Can you work these out from the model? Positions are in its coordinate system, mm. Give positions to 0.01 mm unless a question says otherwise; leave off trailing zeros. Order: outer loops, then holes, each group sorted by start corner. A loop starts at its lowest first (then second) coordinate and runs counter-clockwise, first axis right, second up. Notation, with made-up numbers: M -2.5,47 L 42.5,47 A23 ccw 42.5,78 Z; hole C 36.5,-21 d10. An arc over 180 degrees is marked long. One line per question, with ' | ' between items. Start each with the question number.
1) If we section it at A-A, the plane x = 0.7: State how many separate pieces and enclosed holes the cut face has, plus the area to 3 significant figures.
2) Please list where these lines run through material, in increasing order: line 1 along Z through (x, y) = (1.5, 95.25) (3 decimals); line 2 along Y through (x, z) = (1.35, 0) (3 decimals); line 3 along Z through (x, y) = (1.2, 104.75) (3 decimals). Write a range as [from, to].
3) If we section it at B-B, the plane z = -34.5: Please give me the cut outline in (x, y) (3 decimals).
4) I'm going to push flat-ended pins straight in: pin 1 Ø3.5 at (y, z) = (95.25, 9.5) entering from -X; pin 2 Ø1.6 at (x, y) = (1, 98.5) entering from +Z (3 decimals); pin 3 Ø1.6 at (x, z) = (1, 43) entering from -Y; pin 4 Ø1.6 at (x, z) = (1.5, 45) entering from +Y. Where does each tip first touch, or does it pass through?
```python
from build123d import *

# Parameters (mm, degrees)
SKETCH1_W               = 95.25
SKETCH1_H               = 311.15
BOSS_EXTRUDE1_DEPTH     = 3.175
SKETCH2_W               = 12.7
SKETCH2_H               = 3.175
SKETCH2_W_2             = 19.05
CUT_EXTRUDE1_DEPTH      = 3.175
SKETCH3_W               = 6.35
SKETCH3_H               = 10.16
CUT_EXTRUDE2_DEPTH      = 3.175
MIRROR3_COPY_1_SKETCH_W = 6.35
MIRROR3_COPY_1_SKETCH_H = 10.16
MIRROR3_COPY_1_DEPTH    = 3.175
CUT_EXTRUDE3_DEPTH      = 3.175


with BuildPart() as part:
    # Sketch1 → Boss-Extrude1 (new body)
    with BuildSketch(Plane(origin=(0, 0, 0), x_dir=(0, 0, -1), z_dir=(1, 0, 0))):
        Rectangle(SKETCH1_W, SKETCH1_H)
    extrude(amount=BOSS_EXTRUDE1_DEPTH)

    # Sketch2 → Cut-Extrude1 (cut)
    with BuildSketch(Plane(origin=(3.175, 0, 0), x_dir=(0, 0, -1), z_dir=(1, 0, 0))):
        with Locations((9.525, -153.9875)):
            Rectangle(SKETCH2_W, SKETCH2_H)
        with Locations((-15.875, -153.9875)):
            Rectangle(SKETCH2_W, SKETCH2_H)
        with Locations((-41.275, -153.9875)):
            Rectangle(SKETCH2_W, SKETCH2_H)
        with Locations((38.1, -153.9875)):
            Rectangle(SKETCH2_W_2, SKETCH2_H)
    cut_extrude1 = extrude(amount=-CUT_EXTRUDE1_DEPTH, mode=Mode.SUBTRACT)

    # Mirror1: Cut-Extrude1 across plane
    add(cut_extrude1.mirror(Plane.ZX), mode=Mode.SUBTRACT)

    # Sketch3 → Cut-Extrude2 (cut)
    with BuildSketch(Plane(origin=(3.175, 0, 0), x_dir=(0, 0, -1), z_dir=(1, 0, 0))):
        with Locations((44.45, 96.52)):
            Rectangle(SKETCH3_W, SKETCH3_H)
        with Locations((44.45, 76.2)):
            Rectangle(SKETCH3_W, SKETCH3_H)
        with Locations((44.45, 55.88)):
            Rectangle(SKETCH3_W, SKETCH3_H)
    cut_extrude2 = extrude(amount=-CUT_EXTRUDE2_DEPTH, mode=Mode.SUBTRACT)

    # Mirror2: Cut-Extrude2 across plane
    add(cut_extrude2.mirror(Plane.XY), mode=Mode.SUBTRACT)

    # Mirror3: Cut-Extrude2 across plane
    add(cut_extrude2.mirror(Plane.ZX), mode=Mode.SUBTRACT)

    # Mirror3 copy 1 sketch → Mirror3 copy 1 (cut)
    with BuildSketch(Plane(origin=(3.175, 0, 0), x_dir=(0, 0, 1), z_dir=(1, 0, 0))):
        with Locations((44.45, 96.52)):
            Rectangle(MIRROR3_COPY_1_SKETCH_W, MIRROR3_COPY_1_SKETCH_H)
        with Locations((44.45, 76.2)):
            Rectangle(MIRROR3_COPY_1_SKETCH_W, MIRROR3_COPY_1_SKETCH_H)
        with Locations((44.45, 55.88)):
            Rectangle(MIRROR3_COPY_1_SKETCH_W, MIRROR3_COPY_1_SKETCH_H)
    extrude(amount=-MIRROR3_COPY_1_DEPTH, mode=Mode.SUBTRACT)

    # Sketch5 → Cut-Extrude3 (cut)
    with BuildSketch(Plane(origin=(3.175, 0, 0), x_dir=(0, 0, -1), z_dir=(1, 0, 0))):
        with BuildLine():
            Line((1.060660172, 103.689339828), (0, 104.75))
            Line((0, 104.75), (-1.060660172, 103.689339828))
            ThreePointArc((-1.060660172, 103.689339828), (0, 103.25), (1.060660172, 103.689339828))
        make_face()
        with BuildLine():
            Line((-1.060660172, 103.689339828), (0, 104.75))
            Line((0, 104.75), (1.060660172, 103.689339828))
            ThreePointArc((1.060660172, 103.689339828), (1.385819299, 104.175974851), (1.5, 104.75))
            ThreePointArc((1.5, 104.75), (-0.574025149, 106.135819299), (-1.060660172, 103.689339828))
        make_face()
        with BuildLine():
            ThreePointArc((11, 95.25), (10.074025149, 96.635819299), (8.439339828, 96.310660172))
            Line((8.439339828, 96.310660172), (9.5, 95.25))
            Line((9.5, 95.25), (8.439339828, 94.189339828))
            ThreePointArc((8.439339828, 94.189339828), (10.074025149, 93.864180701), (11, 95.25))
        make_face()
        with BuildLine():
            Line((9.5, 95.25), (8.439339828, 96.310660172))
            ThreePointArc((8.439339828, 96.310660172), (8, 95.25), (8.439339828, 94.189339828))
            Line((8.439339828, 94.189339828), (9.5, 95.25))
        make_face()
        with BuildLine():
            ThreePointArc((-8, 95.25), (-8.114180701, 95.824025149), (-8.439339828, 96.310660172))
            Line((-8.439339828, 96.310660172), (-9.5, 95.25))
            Line((-9.5, 95.25), (-8.439339828, 94.189339828))
            ThreePointArc((-8.439339828, 94.189339828), (-8.114180701, 94.675974851), (-8, 95.25))
        make_face()
        with BuildLine():
            Line((-9.5, 95.25), (-8.439339828, 96.310660172))
            ThreePointArc((-8.439339828, 96.310660172), (-11, 95.25), (-8.439339828, 94.189339828))
            Line((-8.439339828, 94.189339828), (-9.5, 95.25))
        make_face()
        with BuildLine():
            ThreePointArc((1.060660172, 86.810660172), (0, 87.25), (-1.060660172, 86.810660172))
            Line((-1.060660172, 86.810660172), (0, 85.75))
            Line((0, 85.75), (1.060660172, 86.810660172))
        make_face()
        with BuildLine():
            Line((0, 85.75), (-1.060660172, 86.810660172))
            ThreePointArc((-1.060660172, 86.810660172), (-0.574025149, 84.364180701), (1.5, 85.75))
            ThreePointArc((1.5, 85.75), (1.385819299, 86.324025149), (1.060660172, 86.810660172))
            Line((1.060660172, 86.810660172), (0, 85.75))
        make_face()
    extrude(amount=-CUT_EXTRUDE3_DEPTH, mode=Mode.SUBTRACT)


solid = part.part
```
Results found:
1) separate pieces: 1 | enclosed holes: 4 | area: 28,500 mm²
2) line 1: z = [-41.275, -11], [-8, 8], [11, 41.275] | line 2: y = [-155.575, 84.25], [87.25, 103.25], [106.25, 155.575] | line 3: z = [-47.625, -1.5], [1.5, 47.625]
3) outline: M 0,-152.4 L 3.175,-152.4 L 3.175,152.4 L 0,152.4 Z
4) pin 1: stops at x = 0 | pin 2: stops at z = 41.275 | pin 3: stops at y = -152.4 | pin 4: stops at y = 152.4
